from build123d import *

# Parameters (mm, degrees)
SKETCH1_W           = 240
SKETCH1_H           = 60
BOSS_EXTRUDE1_DEPTH = 5
SKETCH2_W           = 10
SKETCH2_H           = 60
BOSS_EXTRUDE2_DEPTH = 20
SKETCH3_R           = 5
BOSS_EXTRUDE3_DEPTH = 230


with BuildPart() as part:
    # Sketch1 → Boss-Extrude1 (new body)
    with BuildSketch(Plane(origin=(0, 0, 0), x_dir=(1, 0, 0), z_dir=(0, 1, 0))):
        Rectangle(SKETCH1_W, SKETCH1_H)
    extrude(amount=BOSS_EXTRUDE1_DEPTH)

    # Sketch2 → Boss-Extrude2 (add)
    with BuildSketch(Plane(origin=(0, 5, 0), x_dir=(1, 0, 0), z_dir=(0, 1, 0))):
        with Locations((-115, 0)):
            Rectangle(SKETCH2_W, SKETCH2_H)
    extrude(amount=BOSS_EXTRUDE2_DEPTH)

    # Sketch3 → Boss-Extrude3 (add, through all)
    with BuildSketch(Plane(origin=(-110, 0, 0), x_dir=(0, 0, -1), z_dir=(1, 0, 0))):
        with Locations(Location((0, 14.27, 0), (0, 0, 180))):
            Circle(SKETCH3_R)
    extrude(amount=BOSS_EXTRUDE3_DEPTH)


solid = part.part
Input: part model. Units: mm. Frame: model coordinates. Round coordinates to 2 decimals unless told otherwise and drop trailing zeros. Loops run counter-clockwise (first coordinate to the right, second up) from the corner with the lowest first, then second, coordinate; pieces in that order, holes last. Notation, with made-up numbers: M 7,6 L 59,6 A17 ccw 59,23 Z; hole C 54,49 d10. An arc over 180 degrees is marked long. Answer as CSV lines item,"result". Start each with the question number.
(1) Line query: line 1 (Y direction, x = 4.5, z = 14.5); line 2 (Y direction, x = 52, z = 0); line 3 (X direction, y = 7.5, z = 24). Output: solid intervals per line, ascending. Write a range as [from, to].
(2) Section A-A, the plane x = 50.5. Output: boundary loops of the cut face in (y, z), plus the area to 3 significant figures.
(3) First-contact query: pin 1 (10 mm diameter, centred on y = 12.5, z = 12, fed in from +X); pin 2 (1 mm diameter, centred on x = -90.5, z = 21.5, fed in from +Y); pin 3 (8 mm diameter, centred on x = -20.5, y = 22, fed in from -Z). Flat tips, straight axial feed; report the tip coordinate or a pass-through.
(4) Section B-B, the plane y = 14.27. Output: boundary loops of the cut face in (x, z).
(5) Draft query along Y for faces 1 (the flat face through (-18, 4, -30)), 2 (the cylindrical face through (3.39, 9.313, -0.651)), 3 (the flat face through (-115, 25, 0)). Return one class per face: released by +Y, released by -Y, zero draft, split by the parting line, or undercut.
(6) Section C-C, the plane z = 0. Output: boundary loops of the cut face in (x, y), plus the area to 3 significant figures.
(7) Section D-D, the plane z = 17.5. Output: boundary loops of the cut face in (x, y).
Values found:
1,line 1,"y = [0, 5]"
1,line 2,"y = [0, 5], [9.27, 19.27]"
1,line 3,"x = [-120, -110]"
2,outline,"M 0,-30 L 5,-30 L 5,30 L 0,30 Z; C 14.27,0 d10"
2,area,"379 mm²"
3,pin 1,"stops at x = -110"
3,pin 2,"stops at y = 5"
3,pin 3,"stops at z = -3.33"
4,outline,"M -120,-30 L -110,-30 L -110,-5 L 120,-5 L 120,5 L -110,5 L -110,30 L -120,30 Z"
5,face 1,"zero draft"
5,face 2,"undercut"
5,face 3,"released by +Y"
6,outline,"M -120,0 L 120,0 L 120,5 L -110,5 L -110,9.27 L 120,9.27 L 120,19.27 L -110,19.27 L -110,25 L -120,25 Z"
6,area,"3,700 mm²"
7,outline,"M -120,0 L 120,0 L 120,5 L -110,5 L -110,25 L -120,25 Z"
